from build123d import *

# Parameters (mm, degrees)
EXTRUDE_1_DEPTH = 47
EXTRUDE_3_DEPTH = 1


with BuildPart() as part:
    # 草图1 → 凸台-拉伸1 (new body)
    with BuildSketch(Plane(origin=(0, 0, 0), x_dir=(1, 0, 0), z_dir=(0, 1, 0))):
        Polygon((-23, 2.1), (23, 2.1), (23, 1.1), (22, 1.1), (23, 0.1), (22, 0.1), (21, 1.1), (-21, 1.1), (-22, 0.1), (-23, 0.1), (-22, 1.1), (-23, 1.1), align=None)
    extrude(amount=EXTRUDE_1_DEPTH)

    # 草图2 → 凸台-拉伸3 (add)
    with BuildSketch(Plane.XZ):
        Polygon((22, -0.1), (-22, -0.1), (-21, -1.1), (21, -1.1), align=None)
    extrude(amount=-EXTRUDE_3_DEPTH)


solid = part.part
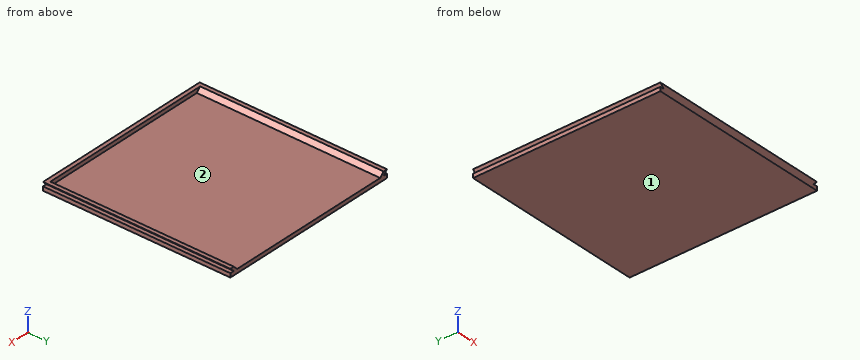
CAD build for the part. Positions are in the model's coordinates, mm. Face numbers are marked on the shaded views. Coordinates: 2 decimals unless noted, no trailing zeros. Order: outer loops, then holes, each group sorted by start corner. A loop starts at its lowest first (then second) coordinate and runs counter-clockwise, first axis right, second up.
Item 1: Drill centre lines: L1, parallel to Z at x = 16, y = 23; L2, parallel to Y at x = -16, z = -0.8; L3, parallel to X at y = 28.5, z = -0.85. Where is each one in solid material? Low to high.
Check sheet entries:
L1: z = -2.1 to -1.1
L2: y = 0 to 1
L3: x = -22.25 to -21.25, 21.25 to 22.25
Item 2: Two-plate mould, pull along X, no slides. Class the marked faces 1 and 2: +X half, -X half, draft (parallel to the pull), parting line (faces both ways), or undercut.
Check sheet entries:
face 1: draft
face 2: undercut
Item 3: Pin check, flat tips, straight feed: pin 1 Ø10 at (x, y) = (12.5, 21.5) entering from +Z; pin 2 Ø1.1 at (x, z) = (6.5, -0.5) entering from +Y. Stop position of each tip, or through.
Check sheet entries:
pin 1: stops at z = -1.1
pin 2: stops at y = 1
Item 4: Band-saw the part on A-A on y = 34. List the corners of the cut face in (x, z).
Check sheet entries:
outline: (-23, -2.1) - (23, -2.1) - (23, -1.1) - (22, -1.1) - (23, -0.1) - (22, -0.1) - (21, -1.1) - (-21, -1.1) - (-22, -0.1) - (-23, -0.1) - (-22, -1.1) - (-23, -1.1) - close
Item 5: Band-saw the part on C-C on x = 14.5. List the corners of the cut face in (y, z), plus the area to 3 significant figures.
Check sheet entries:
outline: (0, -2.1) - (47, -2.1) - (47, -1.1) - (1, -1.1) - (1, -0.1) - (0, -0.1) - close
area: 48.0 mm2
Item 6: Band-saw the part on B-B on z = -0.4. List the corners of the cut face in (x, y), plus the area to 3 significant figures.
Check sheet entries:
outline: (-22.7, 0) - (22.7, 0) - (22.7, 47) - (21.7, 47) - (21.7, 1) - (-21.7, 1) - (-21.7, 47) - (-22.7, 47) - close
area: 137 mm2
